Could you check a few things on this model? Use its own coordinates, in mm. Face numbers are marked on the shaded views. A direction names the side the tool comes from. Coordinates: 2 decimals unless noted, no trailing zeros. Loops run counter-clockwise (first coordinate to the right, second up) from the corner with the lowest first, then second, coordinate; pieces in that order, holes last. Notation, with made-up numbers: (46, 12.5) - (95, 12.5) arc R29 cw to (95, 40.5) - close; hole circle Ø2 at (24.25, 10). An arc over 180 degrees is marked (long way). One line per question, with ' | ' between items. Start each with the question number.
1. Which directions (+Z, -Z, +X, -X, +Y, -Y) give clear straight access to the entire face, cutting with the end or side of a thin tool? Please do the marked faces 4 and 5.
2. Please list where these lines run through material, in increasing order: L1, parallel to Z at x = 48, y = 14.5; L2, parallel to Y at x = 33.5, z = -11; L3, parallel to X at y = 17.75, z = -17. Write a range as [from, to].
3. I want a section at A-A, the plane y = 7.5. Write out the boundary of the cut face in (x, z).
4. I want a section at C-C, the plane x = 14. Write out the boundary of the cut face in (y, z).
5. I'm going to push flat-ended pins straight in: P1, Ø0.6, axis at x = 1, y = 11, coming from the +Z side; P2, Ø4, axis at y = 17, z = -4, coming from the -X side; P3, Ø1, axis at x = 7, z = -8, coming from the +Y side; P4, Ø2, axis at y = 15, z = -15.5, coming from the -X side. Where does each tip first touch, or does it pass through?
6. We'd pull the mould along X, two halves only. Please class the marked faces 1, 2 and 3: pulls with the +X half, pulls with the -X half, needs draft (parallel to the pull), parting line crosses it, or undercut.
7. I want a section at B-B, the plane z = -6. Write out the boundary of the cut face in (x, y).
from build123d import *

# Parameters (mm, degrees)
SKETCH1_W           = 51
SKETCH1_H           = 31
BOSS_EXTRUDE1_DEPTH = 2
SKETCH2_W           = 2
SKETCH2_H           = 1
BOSS_EXTRUDE2_DEPTH = 17
FILLET3_R           = 2
FILLET4_R           = 2
FILLET5_R           = 2
FILLET6_R           = 2


with BuildPart() as part:
    # Sketch1 → Boss-Extrude1 (new body)
    with BuildSketch(Plane(origin=(0, 0, 0), x_dir=(1, 0, 0), z_dir=(0, 1, 0))):
        with Locations((25.5, 15.5)):
            Rectangle(SKETCH1_W, SKETCH1_H)
    extrude(amount=BOSS_EXTRUDE1_DEPTH)

    # Sketch2 → Boss-Extrude2 (add)
    with BuildSketch(Plane(origin=(0, 2, 0), x_dir=(1, 0, 0), z_dir=(0, 1, 0))):
        Polygon((49, 2), (49, 0), (51, 0), (51, 31), (49, 31), (49, 29), align=None)
        Polygon((0, 2), (0, 0), (49, 0), (49, 2), (2, 2), align=None)
        Polygon((2, 29), (49, 29), (49, 31), (0, 31), (0, 29), align=None)
        with Locations((1, 28.5)):
            Rectangle(SKETCH2_W, SKETCH2_H)
        with Locations((1, 2.5)):
            Rectangle(SKETCH2_W, SKETCH2_H)
    extrude(amount=BOSS_EXTRUDE2_DEPTH)

    # Fillet3
    fillet3_edges = [part.edges().sort_by_distance(p)[0] for p in [
        (51, 9.5, 0),
    ]]
    fillet(fillet3_edges, radius=FILLET3_R)

    # Fillet4
    fillet4_edges = [part.edges().sort_by_distance(p)[0] for p in [
        (51, 9.5, -31),
    ]]
    fillet(fillet4_edges, radius=FILLET4_R)

    # Fillet5
    fillet5_edges = [part.edges().sort_by_distance(p)[0] for p in [
        (0, 9.5, 0),
    ]]
    fillet(fillet5_edges, radius=FILLET5_R)

    # Fillet6
    fillet6_edges = [part.edges().sort_by_distance(p)[0] for p in [
        (0, 9.5, -31),
    ]]
    fillet(fillet6_edges, radius=FILLET6_R)


solid = part.part
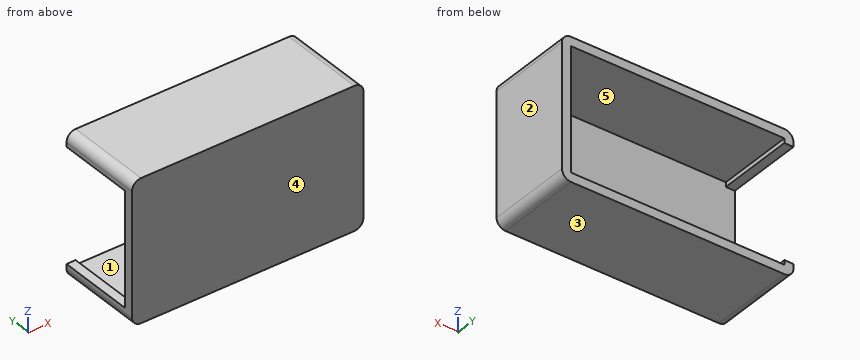
Results are:
1) face 4: +Z, -Z, +X, -X, -Y | face 5: +Y
2) L1: z = [-31, -29], [-2, 0] | L2: y = [0, 2] | L3: x = [49, 51]
3) outline: (0, -29) arc R2 ccw to (2, -31) - (49, -31) arc R2 ccw to (51, -29) - (51, -2) arc R2 ccw to (49, 0) - (2, 0) arc R2 ccw to (0, -2) - (0, -3) - (2, -3) - (2, -2) - (49, -2) - (49, -29) - (2, -29) - (2, -28) - (0, -28) - close
4) outline: (0, -31) - (19, -31) - (19, -29) - (2, -29) - (2, -2) - (19, -2) - (19, 0) - (0, 0) - close
5) P1: stops at z = -0.13 | P2: stops at x = 0 | P3: stops at y = 2 | P4: stops at x = 49
6) face 1: undercut | face 2: pulls with the +X half | face 3: needs draft
7) outline: (0, 0) - (51, 0) - (51, 19) - (49, 19) - (49, 2) - (0, 2) - close
